from build123d import *

# Parameters (mm, degrees)
SKETCH_1_W      = 112
SKETCH_1_H      = 54.2
SKETCH_1_R      = 1.65
EXTRUDE_1_DEPTH = 2


with BuildPart() as part:
    # 草图1 → 凸台-拉伸1 (new body)
    with BuildSketch(Plane(origin=(0, 0, 0), x_dir=(1, 0, 0), z_dir=(0, 1, 0))):
        with Locations((56, -27.1)):
            Rectangle(SKETCH_1_W, SKETCH_1_H)
        with Locations(Location((5, -5, 0), (0, 0, 270))):
            Circle(SKETCH_1_R, mode=Mode.SUBTRACT)
        with Locations(Location((107, -5, 0), (0, 0, 270))):
            Circle(SKETCH_1_R, mode=Mode.SUBTRACT)
        with Locations(Location((107, -49.2, 0), (0, 0, 270))):
            Circle(SKETCH_1_R, mode=Mode.SUBTRACT)
        with Locations(Location((5, -49.2, 0), (0, 0, 270))):
            Circle(SKETCH_1_R, mode=Mode.SUBTRACT)
    extrude(amount=EXTRUDE_1_DEPTH)


solid = part.part
Design review of the part built by this model. Coordinates are the model's own, in mm. Round coordinates to 2 decimals unless told otherwise and drop trailing zeros. Write each loop counter-clockwise with the first axis right and the second up, starting at its lowest first coordinate (ties: lowest second). Pieces come first, ordered by that corner, then holes. Notation, with made-up numbers: M 15.25,11 L 35.25,11 A14 cw 35.25,18 Z; hole C -35,17 d6. An arc over 180 degrees is marked long. One line per item, written item: value. Start each with the question number.
1. Draft analysis for pull direction X (two halves, no side actions). For faces 1 (the face through (55, 2, 27)), 2 (the face through (5.07, 0.99, 47.55)), 3 (the face through (112, 1, 27)), state which applies: pulls with the +X half, pulls with the -X half, needs draft (parallel to the pull), parting line crosses it, or undercut.
2. Take a section at A-A on x = 107. State the section outline as (y, z) points.
3. To check wall thickness, follow probe 1 along Z at (x, y) = (107, 0.9); probe 2 along X at (y, z) = (1.05, 49.2); probe 3 along X at (y, z) = (1.25, 50.5). State the ranges of each line that lie inside material, in increasing order. Write a range as from..to.
4. Clearance check with flat-ended pins moving along their axes: P1, Ø4.5, axis at x = 5, z = 49.2, coming from the +Y side; P2, Ø2, axis at x = 107, z = 5, coming from the -Y side. State where each tip first meets the part, or that it passes through.
Computed:
1. face 1: needs draft
1. face 2: undercut
1. face 3: pulls with the +X half
2. outline: M 0,0 L 2,0 L 2,3.35 L 0,3.35 Z; M 0,6.65 L 2,6.65 L 2,47.55 L 0,47.55 Z; M 0,50.85 L 2,50.85 L 2,54.2 L 0,54.2 Z
3. probe 1: z = 0..3.35, 6.65..47.55, 50.85..54.2
3. probe 2: x = 0..3.35, 6.65..105.35, 108.65..112
3. probe 3: x = 0..3.98, 6.02..105.98, 108.02..112
4. P1: stops at y = 2
4. P2: passes through
